Design review of the part built by this model. Coordinates are the model's own, in mm. A direction names the side the tool comes from. Round coordinates to 2 decimals unless told otherwise and drop trailing zeros. Order: outer loops, then holes, each group sorted by start corner. A loop starts at its lowest first (then second) coordinate and runs counter-clockwise, first axis right, second up. Notation, with made-up numbers: (-23.75, 21) - (7.25, 21) arc R31 ccw to (7.25, 48) - close; hole circle Ø5 at (26, 89). An arc over 180 degrees is marked (long way). Answer as a JSON object with one key per item and string values. Group by question number.
Autodesk Inventor part; units mm, degrees
ref_plane "YZ Plane" through (0, 0, 0) normal (1, 0, 0) x (0, 1, 0)
ref_plane "XZ Plane" through (0, 0, 0) normal (0, 1, 0) x (-1, 0, 0)
ref_plane "XY Plane" through (0, 0, 0) normal (0, 0, 1) x (1, 0, 0)
sketch "Эскиз1" plane through (0, 0, 0) normal (0, 0, 1) x (1, 0, 0)
  line L0 (49.9998, 0) -> (189, 0)
  line L1 (148.768, -39) -> (70.9998, -39)
  line L2 (49.9998, -20) -> (49.9998, 0)
  arc A0 (70.9998, -39) -> (54.9998, -55) centre (70.9998, -55) ccw
  arc A1 (34.9998, -94) -> (24.9998, -84) centre (24.9998, -94) ccw
  line L3 (0, 0) -> (0, 25.6698)
  line L4 (54.9998, -132) -> (54.9998, -55)
  line L5 (189, 0) -> (189, -28)
  line L6 (189, -28) -> (178, -28)
  line L7 (178, -28) -> (178, -108)
  line L8 (178, -108) -> (189, -108)
  line L9 (189, -108) -> (189, -120)
  line L10 (189, -120) -> (178, -120)
  line L11 (178, -120) -> (178, -132)
  line L12 (178, -132) -> (189, -132)
  line L13 (189, -132) -> (189, -144)
  line L14 (189, -144) -> (178, -144)
  line L15 (178, -144) -> (178, -156)
  line L16 (24.9998, -84) -> (22.4998, -84)
  line L17 (22.4998, -84) -> (22.4998, -20)
  line L18 (22.4998, -20) -> (49.9998, -20)
  line L19 (34.9998, -94) -> (34.9998, -156)
  line L20 (34.9998, -156) -> (39.9998, -156)
  line L21 (39.9998, -156) -> (39.9998, -148)
  line L22 (39.9998, -148) -> (54.9998, -148)
  line L23 (54.9998, -148) -> (54.9998, -132)
  line L24 (178, -156) -> (169, -156)
  line L25 (169, -156) -> (169, -148)
  line L26 (169, -148) -> (160, -148)
  line L27 (160, -148) -> (160, -86)
  line L28 (160, -86) -> (164.566, -57.5341)
  arc A2 (164.566, -57.5341) -> (148.768, -39) centre (148.768, -55) ccw
  point P0 (154.5118, -39)
  point P1 (54.9998, -39)
  point P2 (34.9998, -84)
  point P3 (137.0508, -39)
  dimension "d0" = 189
  dimension "d5" = 99.512
  dimension "d9" = 16
  dimension "d11" = 10
  dimension "d29" = 20
  dimension "d30" = 28
  dimension "d31" = 11
  dimension "d32" = 80
  dimension "d34" = 12
  dimension "d35" = 11
  dimension "d36" = 12
  dimension "d37" = 11
  dimension "d38" = 12
  dimension "d39" = 11
  dimension "d40" = 12
  dimension "d43" = 2.5
  dimension "d44" = 64
  dimension "d45" = 15
  dimension "d46" = 8
  dimension "d47" = 5
  dimension "d50" = 9
  dimension "d51" = 9
  dimension "d52" = 16
revolve "Вращение1" add sketch "Эскиз1" angle 360 about axis through (0, 0, 0) along (0, 1, 0)
properties part number "Нижняя часть поршня_CPY" material "Чугун, серый"
1. To check wall thickness, follow line 1 (Z direction, x = 0, y = -110.5); line 2 (Z direction, x = 0, y = -98); line 3 (X direction, y = -153.5, z = 0). State the ranges of each line that lie inside material, in increasing order. Write a range as from..to.
2. Clearance check with flat-ended pins moving along their axes: P1, Ø2, axis at x = -124, y = -42, coming from the +Z side; P2, Ø5, axis at y = -72.5, z = 138.5, coming from the +X side; P3, Ø1, axis at y = -113.5, z = -43, coming from the -X side. State where each tip first meets the part, or that it passes through.
3. Take a section at B-B, the plane y = -50.5. Give the boundary of the cut face in (x, z), then the cut area to 3 significant figures.
4. Take a section at A-A, the plane y = -102. Give the boundary of the cut face in (x, z).
5. Mouldability with a two-part tool opening along X and no side actions: class faces 1 (the flat face through (-0.2, -156, 35.4)), 2 (the cylindrical face through (33.384, -125.434, 10.513)), 3 (the cylindrical face through (-149.984, -138.084, -115.004)) as pulls with the +X half, pulls with the -X half, needs draft (parallel to the pull), parting line crosses it, or undercut.
6. Tool access review of faces 4 (the flat face through (-127, -120, 125)), 5 (the cylindrical face through (-149.984, -114.084, -115.004)), 6 (the cylindrical face through (-7.16, -100.85, -54.53)), 7 (the flat face through (22, -20, 10)): name each direction out of +Z, -Z, +X, -X, +Y, -Y from which nothing blocks a thin tool from reaching the whole face with its end or side.
Response values:
{
 "1": {"line 1": "-189..-160, -55..-35, 35..55, 160..189", "line 2": "-178..-160, -55..-35, 35..55, 160..178", "line 3": "-178..-169, -40..-35, 35..40, 169..178"},
 "2": {"P1": "z = 128.67", "P2": "x = 114.84", "P3": "x = -184.16"},
 "3": {"outline": "circle Ø356 at (0, 0); circle Ø111.29 at (0, 0); hole circle Ø328.24 at (0, 0); hole circle Ø45 at (0, 0)", "area": "23,100 mm2"},
 "4": {"outline": "circle Ø356 at (0, 0); circle Ø110 at (0, 0); hole circle Ø320 at (0, 0); hole circle Ø70 at (0, 0)"},
 "5": {"face 1": "needs draft", "face 2": "undercut", "face 3": "parting line crosses it"},
 "6": {"face 4": "none", "face 5": "+Y, -Y", "face 6": "-Y", "face 7": "+Y"}
}
